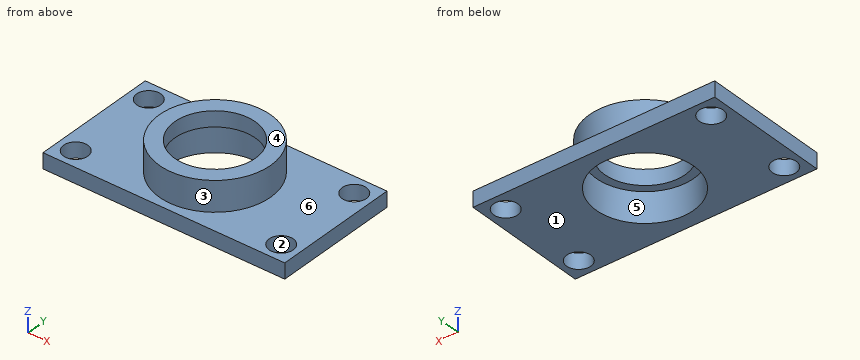
from build123d import *

# Parameters (mm, degrees)
SKETCH2_W           = 40
SKETCH2_H           = 21
BOSS_EXTRUDE1_DEPTH = 2.54
SKETCH4_R           = 9.2075
BOSS_EXTRUDE2_DEPTH = 4.9784
CUT_EXTRUDE2_START  = 7.5184
SKETCH7_R           = 6.6675
CUT_EXTRUDE2_DEPTH  = 2.54
SKETCH8_R           = 1.999996
CUT_EXTRUDE3_DEPTH  = 3.54
SKETCH10_R          = 1.999996
CUT_EXTRUDE4_DEPTH  = 3.54
SKETCH13_R          = 8.0645
CUT_EXTRUDE5_DEPTH  = 4.9784


with BuildPart() as part:
    # Sketch2 → Boss-Extrude1 (new body)
    with BuildSketch(Plane.XY):
        with Locations((20, 10.5)):
            Rectangle(SKETCH2_W, SKETCH2_H)
    extrude(amount=BOSS_EXTRUDE1_DEPTH)

    # Sketch4 → Boss-Extrude2 (add)
    with BuildSketch(Plane.XY.offset(2.54)):
        with Locations((20.0000108, 10.49999932)):
            Circle(SKETCH4_R)
    extrude(amount=BOSS_EXTRUDE2_DEPTH)

    # Sketch7 → Cut-Extrude2 (cut)
    with BuildSketch(Plane.XY.offset(CUT_EXTRUDE2_START)):
        with Locations((20.0000108, 10.49999932)):
            Circle(SKETCH7_R)
    extrude(amount=-CUT_EXTRUDE2_DEPTH, mode=Mode.SUBTRACT)

    # Sketch8 → Cut-Extrude3 (cut, through all)
    with BuildSketch(Plane.XY.offset(2.54)):
        with Locations((37.000006, 18.000006)):
            Circle(SKETCH8_R)
        with Locations((3.0000156, 18.000006)):
            Circle(SKETCH8_R)
    extrude(amount=-CUT_EXTRUDE3_DEPTH, mode=Mode.SUBTRACT)

    # Sketch10 → Cut-Extrude4 (cut, through all)
    with BuildSketch(Plane.XY.offset(2.54)):
        with Locations((37.000006, 2.999994)):
            Circle(SKETCH10_R)
        with Locations((3.0000156, 2.999994)):
            Circle(SKETCH10_R)
    extrude(amount=-CUT_EXTRUDE4_DEPTH, mode=Mode.SUBTRACT)

    # Sketch13 → Cut-Extrude5 (cut)
    with BuildSketch(Plane(origin=(0, 0, 0), x_dir=(-1, 0, 0), z_dir=(0, 0, -1))):
        with Locations((-19.9999892, 10.49999932)):
            Circle(SKETCH13_R)
    extrude(amount=-CUT_EXTRUDE5_DEPTH, mode=Mode.SUBTRACT)


solid = part.part
For this review, take the finished solid that the model builds, in its own axes (mm). Face numbers are marked on the shaded views. A direction names the side the tool comes from. Coordinates: 2 decimals unless noted, no trailing zeros. Order: outer loops, then holes, each group sorted by start corner. A loop starts at its lowest first (then second) coordinate and runs counter-clockwise, first axis right, second up. Notation, with made-up numbers: (20.25, 32) -> (37.25, 32) arc R10 ccw to (37.25, 44) -> close; hole circle Ø10 at (18, -19). An arc over 180 degrees is marked (long way). Return JSON: item names as keys, results as strings.
1. We need section B-B on x = 24. Write out the cut boundary in (y, z).
Answer block:
{"outline": "(0, 0) -> (3.5, 0) -> (3.5, 4.98) -> (5.17, 4.98) -> (5.17, 7.52) -> (2.21, 7.52) -> (2.21, 2.54) -> (0, 2.54) -> close; (15.83, 4.98) -> (17.5, 4.98) -> (17.5, 0) -> (21, 0) -> (21, 2.54) -> (18.79, 2.54) -> (18.79, 7.52) -> (15.83, 7.52) -> close"}
2. Machinability: for the marked faces 4, 5 and 6, which of the approach directions +Z, -Z, +X, -X, +Y, -Y give a long, thin tool a straight path to every point of the face, cutting with its end or side? Answer none if there is none.
Answer block:
{"face 4": "+Z, +X, -X, +Y, -Y", "face 5": "-Z", "face 6": "+Z"}
3. The part is to be moulded in two halves that separate along X. For the marked faces 1, 2 and 3, say which applies: +X half, -X half, draft (parallel to the pull), parting line (faces both ways), or undercut.
Answer block:
{"face 1": "draft", "face 2": "undercut", "face 3": "parting line"}
4. We need section C-C on z = 4.5. Write out the cut boundary in (x, y) (1 decimal).
Answer block:
{"outline": "circle Ø18.4 at (20, 10.5); hole circle Ø16.1 at (20, 10.5)"}
5. For line 1 (Y direction, x = 37, z = 1); line 2 (Y direction, x = 36, z = 0.5); line 3 (X direction, y = 2, z = 0.75), list the stretches that pass through material, from the lowest coordinate up. Write a range as from..to.
Answer block:
{"line 1": "0..1, 5..16, 20..21", "line 2": "0..1.27, 4.73..16.27, 19.73..21", "line 3": "0..1.27, 4.73..35.27, 38.73..40"}
6. We need section A-A on y = 10.5. Write out the cut boundary in (x, z).
Answer block:
{"outline": "(0, 0) -> (11.94, 0) -> (11.94, 4.98) -> (13.33, 4.98) -> (13.33, 7.52) -> (10.79, 7.52) -> (10.79, 2.54) -> (0, 2.54) -> close; (26.67, 4.98) -> (28.06, 4.98) -> (28.06, 0) -> (40, 0) -> (40, 2.54) -> (29.21, 2.54) -> (29.21, 7.52) -> (26.67, 7.52) -> close"}
7. For pin 1 Ø5 at (x, y) = (3, 3) entering from +Z; pin 2 Ø1 at (x, z) = (20, 6) entering from +Y; pin 3 Ø2 at (y, z) = (6, 4.5) entering from +X; pin 4 Ø3.5 at (x, y) = (37, 3) entering from -Z, all flat-tipped, find the tip position at first contact; note any pin that passes through.
Answer block:
{"pin 1": "z = 2.54", "pin 2": "y = 19.71", "pin 3": "x = 28.52", "pin 4": "through"}
